Autodesk Inventor part; units mm, degrees
ref_plane "YZ Plane" through (0, 0, 0) normal (1, 0, 0) x (0, 1, 0)
ref_plane "XZ Plane" through (0, 0, 0) normal (0, 1, 0) x (-1, 0, 0)
ref_plane "XY Plane" through (0, 0, 0) normal (0, 0, 1) x (1, 0, 0)
sketch "草圖1" plane through (0, 0, 0) normal (0, 0, 1) x (1, 0, 0)
  line L0 (5.85, -3.3775) -> (0, -6.755)
  line L1 (5.85, 3.3775) -> (5.85, -3.3775)
  line L2 (0, 6.755) -> (5.85, 3.3775)
  line L3 (-5.85, 3.3775) -> (0, 6.755)
  line L4 (-5.85, -3.3775) -> (-5.85, 3.3775)
  line L5 (0, -6.755) -> (-5.85, -3.3775)
  line L6 (-5.85, 3.3775) -> (0, 6.755)
  line L7 (0, 6.755) -> (5.85, 3.3775)
  line L8 (0, 6.755) -> (5.85, 3.3775)
  line L9 (5.85, 3.3775) -> (7.1, 5.5426)
  line L10 (7.1, 5.5426) -> (1.25, 8.9201)
  line L11 (1.25, 8.9201) -> (0, 6.755)
  line L12 (-5.85, -3.3775) -> (-5.85, 3.3775)
  line L13 (-5.85, 3.3775) -> (-8.35, 3.3775)
  line L14 (-8.35, 3.3775) -> (-8.35, -3.3775)
  line L15 (-8.35, -3.3775) -> (-5.85, -3.3775)
  line L16 (5.85, -3.3775) -> (0, -6.755)
  line L17 (0, -6.755) -> (1.25, -8.9201)
  line L18 (1.25, -8.9201) -> (7.1, -5.5426)
  line L19 (7.1, -5.5426) -> (5.85, -3.3775)
  circle A0 centre (0, 0) radius 16.5
  point P0 (0, -6.755)
  dimension "d2" = 2.5
  dimension "d3" = 360
  dimension "d4" = 33
extrude "擠出1" add sketch "草圖1" along normal blind 3
sketch "草圖2" plane through (0, 0, 3) normal (0, 0, 1) x (1, 0, 0)
  circle A0 centre (0, 0) radius 16.5
  line L0 (0, 6.755) -> (1.25, 8.9201)
  line L1 (1.25, 8.9201) -> (7.1, 5.5426)
  line L2 (7.1, 5.5426) -> (5.85, 3.3775)
  line L3 (5.85, 3.3775) -> (5.85, -3.3775)
  line L4 (5.85, -3.3775) -> (7.1, -5.5426)
  line L5 (7.1, -5.5426) -> (1.25, -8.9201)
  line L6 (1.25, -8.9201) -> (0, -6.755)
  line L7 (0, -6.755) -> (-5.85, -3.3775)
  line L8 (-5.85, -3.3775) -> (-8.35, -3.3775)
  line L9 (-8.35, -3.3775) -> (-8.35, 3.3775)
  line L10 (-8.35, 3.3775) -> (-5.85, 3.3775)
  line L11 (-5.85, 3.3775) -> (0, 6.755)
properties part number "2GTbase"
Can you work these out from the model? Positions are in its coordinate system, mm. A direction names the side the tool comes from. Round coordinates to 2 decimals unless told otherwise and drop trailing zeros. Loops run counter-clockwise (first coordinate to the right, second up) from the corner with the lowest first, then second, coordinate; pieces in that order, holes last. Notation, with made-up numbers: M 28.25,15.25 L 75.25,15.25 A16 ccw 75.25,46.25 Z; hole C 37,58.5 d1. An arc over 180 degrees is marked long. Answer as a JSON object with one key per item and string values. Group by question number.
Q1. Imagine slicing it at C-C, the plane x = -7.5. Please give me the cut outline in (y, z).
Q2. On a 3-axis mill with a long thin cutter (end or side, diameter ignored), from which of +Z, -Z, +X, -X, +Y, -Y can I reach the whole of each face in a straight line? I mean faces 4 (the flat face through (-0.2, -7.1, 0)), 5 (the flat face through (4.134, -7.255, 1.479)). Say none if no direction works.
Q3. Imagine slicing it at A-A, the plane y = 0. Please give me the cut outline in (x, z).
Q4. Imagine slicing it at D-D, the plane y = 11. Please give me the cut outline in (x, z), then the cut area to 3 significant figures.
Q5. Will these pins go through, and if not, where does the flat tip stop? pin 1 (0.8 mm diameter, centred on x = -7, z = 2, fed in from -Y); pin 2 (1.2 mm diameter, centred on x = -7, z = 1.5, fed in from +Y).
Q6. Please list where these lines run through material, in increasing order: L1, parallel to X at y = -1.5, z = 1.1; L2, parallel to Y at x = 2, z = 0.25; L3, parallel to X at y = 3, z = 2.4.
Q7. We'd pull the mould along X, two halves only. Please class faces 1 (the flat face through (4.216, 7.208, 1.479)), 2 (the flat face through (-0.2, -7.1, 3)), 3 (the cylindrical face through (15.24, 6.32, 1.48)): +X half, -X half, draft (parallel to the pull), parting line (faces both ways), or undercut.
Findings:
{
 "1": {"outline": "M -14.7,0 L -3.38,0 L -3.38,3 L -14.7,3 Z; M 3.38,0 L 14.7,0 L 14.7,3 L 3.38,3 Z"},
 "2": {"face 4": "-Z, +X, -X, +Y, -Y", "face 5": "+Z, -Z"},
 "3": {"outline": "M -16.5,0 L -8.35,0 L -8.35,3 L -16.5,3 Z; M 5.85,0 L 16.5,0 L 16.5,3 L 5.85,3 Z"},
 "4": {"outline": "M -12.3,0 L 12.3,0 L 12.3,3 L -12.3,3 Z", "area": "73.8 mm2"},
 "5": {"pin 1": "stops at y = -15.12", "pin 2": "stops at y = 15.21"},
 "6": {"L1": "x = -16.43 to -8.35, 5.85 to 16.43", "L2": "y = -16.38 to -8.49, 8.49 to 16.38", "L3": "x = -16.22 to -8.35, 5.85 to 16.22"},
 "7": {"face 1": "undercut", "face 2": "draft", "face 3": "parting line"}
}
